```python
from build123d import *

# Parameters (mm, degrees)
DODANIE_WYCI_GNI_CIE1_DEPTH = 6
SZKIC3_R                    = 5.05
WYTNIJ_WYCI_GNI_CIE1_DEPTH  = 172.237795034
SZKIC5_R                    = 1.55
SZKIC5_W                    = 26
SZKIC5_H                    = 11
SZKIC5_W_2                  = 16
SZKIC5_H_2                  = 10
WYTNIJ_WYCI_GNI_CIE2_DEPTH  = 172.237795034
DODANIE_WYCI_GNI_CIE2_DEPTH = 6
SZKIC6_R                    = 1.55
WYTNIJ_WYCI_GNI_CIE3_DEPTH  = 172.237795034
DODANIE_WYCI_GNI_CIE3_DEPTH = 6
SZKIC9_R                    = 1.55
WYTNIJ_WYCI_GNI_CIE5_DEPTH  = 6
SZKIC11_R                   = 1.55
WYTNIJ_WYCI_GNI_CIE6_DEPTH  = 6
SZKIC15_R                   = 2.5
WYTNIJ_WYCI_GNI_CIE7_DEPTH  = 6
SZKIC8_R                    = 1.55
WYTNIJ_WYCI_GNI_CIE4_DEPTH  = 172.237795034
SZKIC20_W                   = 6.6
SZKIC20_H                   = 6.6
WYTNIJ_WYCI_GNI_CIE9_DEPTH  = 6
WYTNIJ_WYCI_GNI_CIE10_DEPTH = 10


with BuildPart() as part:
    # Szkic2 → Dodanie-wyciągnięcie1 (new body)
    with BuildSketch(Plane(origin=(0, 0, 0), x_dir=(1, 0, 0), z_dir=(0, 1, 0))):
        with BuildLine():
            Line((-2.705874152, 127.916025414), (-8.705874152, 127.916025414))
            ThreePointArc((-8.705874152, 127.916025414), (-10.120087715, 127.330238976), (-10.705874152, 125.916025414))
            Line((-10.705874152, 125.916025414), (-10.705874152, 88.696086508))
            ThreePointArc((-10.705874152, 88.696086508), (-11.877447027, 85.867659383), (-14.705874152, 84.696086508))
            Line((-14.705874152, 84.696086508), (-30.205874152, 84.696086508))
            ThreePointArc((-30.205874152, 84.696086508), (-33.034301277, 83.524513632), (-34.205874152, 80.696086508))
            Line((-34.205874152, 80.696086508), (-34.205874152, 69.929357434))
            Line((-34.205874152, 69.929357434), (-34.205874152, 68.036244156))
            Line((-34.205874152, 68.036244156), (-34.205874152, 10.604511111))
            Line((-34.205874152, 10.604511111), (-34.205874152, -19.154356935))
            ThreePointArc((-34.205874152, -19.154356935), (-21.880415638, -37.623287954), (-0.095732854, -33.328414665))
            Line((-0.095732854, -33.328414665), (14.157093559, -19.139859884))
            Line((14.157093559, -19.139859884), (55.027168237, 21.545915465))
            ThreePointArc((55.027168237, 21.545915465), (56.334805154, 23.495770338), (56.794125848, 25.798132784))
            Line((56.794125848, 25.798132784), (56.794125848, 30.935818421))
            Line((56.794125848, 30.935818421), (56.794125848, 59.333926751))
            ThreePointArc((56.794125848, 59.333926751), (64.677605901, 81.048439594), (85.935948442, 90.090131813))
            Line((85.935948442, 90.090131813), (91.371133341, 90.090131813))
            ThreePointArc((91.371133341, 90.090131813), (105.458816444, 95.925441216), (111.294125848, 110.013124319))
            Line((111.294125848, 110.013124319), (111.294125848, 128))
            ThreePointArc((111.294125848, 128), (110.70833941, 129.414213562), (109.294125848, 130))
            Line((109.294125848, 130), (103.294125848, 130))
            ThreePointArc((103.294125848, 130), (101.879912285, 129.414213562), (101.294125848, 128))
            Line((101.294125848, 128), (101.294125848, 110))
            ThreePointArc((101.294125848, 110), (98.36519366, 102.928932188), (91.294125848, 100))
            Line((91.294125848, 100), (9.294125848, 100))
            ThreePointArc((9.294125848, 100), (2.223058036, 102.928932188), (-0.705874152, 110))
            Line((-0.705874152, 110), (-0.705874152, 125.916025414))
            ThreePointArc((-0.705874152, 125.916025414), (-1.29166059, 127.330238976), (-2.705874152, 127.916025414))
        make_face()
    extrude(amount=DODANIE_WYCI_GNI_CIE1_DEPTH)

    # Szkic3 → Wytnij-wyciągnięcie1 (cut, through all)
    with BuildSketch(Plane(origin=(0, 6, 0), x_dir=(1, 0, 0), z_dir=(0, 1, 0))):
        with Locations(Location((-13.29618586, -25.303913492, 0), (0, 0, 270))):
            Circle(SZKIC3_R)
    extrude(amount=-WYTNIJ_WYCI_GNI_CIE1_DEPTH, mode=Mode.SUBTRACT)

    # Szkic5 → Wytnij-wyciągnięcie2 (cut, through all)
    with BuildSketch(Plane(origin=(0, 6, 0), x_dir=(1, 0, 0), z_dir=(0, 1, 0))):
        with Locations(Location((40.894125848, 75.45, 0), (0, 0, 270))):
            Circle(SZKIC5_R)
        with Locations(Location((30.260526652, 95, 0), (0, 0, 270))):
            Circle(SZKIC5_R)
        with Locations(Location((6.360542819, 95, 0), (0, 0, 270))):
            Circle(SZKIC5_R)
        with Locations(Location((40.894125848, 46.55, 0), (0, 0, 270))):
            Circle(SZKIC5_R)
        with Locations(Location((17.894125848, 72, 0), (0, 0, 270))):
            Circle(SZKIC5_R)
        with Locations((10.894125848, 52.5)):
            Rectangle(SZKIC5_W, SZKIC5_H)
        with Locations((15.894125848, 85)):
            Rectangle(SZKIC5_W_2, SZKIC5_H_2)
    extrude(amount=-WYTNIJ_WYCI_GNI_CIE2_DEPTH, mode=Mode.SUBTRACT)

    # Szkic12 → Dodanie-wyciągnięcie2 (add)
    with BuildSketch(Plane.XZ):
        with BuildLine():
            Line((28.406352316, 21.766792401), (22.674893132, 30.029606522))
            ThreePointArc((22.674893132, 30.029606522), (15.741620567, 36.230120828), (6.753517107, 38.623996834))
            Line((6.753517107, 38.623996834), (-1.505533921, 38.835570804))
            Line((-1.505533921, 38.835570804), (-13.693695858, 39.147797694))
            Line((-13.693695858, 39.147797694), (55.027168237, -21.545915465))
            ThreePointArc((55.027168237, -21.545915465), (56.334805154, -23.495770338), (56.794125848, -25.798132784))
            Line((56.794125848, -25.798132784), (56.794125848, -59.333926751))
            ThreePointArc((56.794125848, -59.333926751), (64.677605901, -81.048439594), (85.935948442, -90.090131813))
            Line((85.935948442, -90.090131813), (91.371133341, -90.090131813))
            Line((91.371133341, -90.090131813), (111.294125848, -110.013124319))
            Line((111.294125848, -110.013124319), (111.294125848, -103.986622655))
            ThreePointArc((111.294125848, -103.986622655), (110.381700995, -98.014648527), (107.72767835, -92.58757216))
            Line((107.72767835, -92.58757216), (89.166132072, -65.828137643))
            Line((89.166132072, -65.828137643), (62.775344571, -27.781601032))
            Line((62.775344571, -27.781601032), (28.406352316, 21.766792401))
        make_face()
    extrude(amount=-DODANIE_WYCI_GNI_CIE2_DEPTH)

    # Szkic6 → Wytnij-wyciągnięcie3 (cut, through all)
    with BuildSketch(Plane.XZ):
        with Locations(Location((68.241593591, -68.382704099, 0), (0, 0, 270))):
            Circle(SZKIC6_R)
    extrude(amount=-WYTNIJ_WYCI_GNI_CIE3_DEPTH, mode=Mode.SUBTRACT)

    # Szkic13 → Dodanie-wyciągnięcie3 (add)
    with BuildSketch(Plane.XZ):
        with BuildLine():
            Line((-34.205874152, -80.696086508), (-34.205874152, -90.183506419))
            ThreePointArc((-34.205874152, -90.183506419), (-33.840904211, -92.57229607), (-32.779295153, -94.743126617))
            Line((-32.779295153, -94.743126617), (-10.365682355, -127.055930463))
            ThreePointArc((-10.365682355, -127.055930463), (-9.649740147, -127.688003136), (-8.722327105, -127.916025414))
            Line((-8.722327105, -127.916025414), (-6.264571206, -127.916025414))
            Line((-6.264571206, -127.916025414), (-6.264571206, -80.696086508))
            Line((-6.264571206, -80.696086508), (-8.705874152, -80.696086508))
            Line((-8.705874152, -80.696086508), (-34.205874152, -80.696086508))
        make_face()
    extrude(amount=-DODANIE_WYCI_GNI_CIE3_DEPTH)

    # Szkic9 → Wytnij-wyciągnięcie5 (cut)
    with BuildSketch(Plane.XZ):
        with Locations(Location((63.668699873, -36.96490988, 0), (0, 0, 270))):
            Circle(SZKIC9_R)
    extrude(amount=-WYTNIJ_WYCI_GNI_CIE5_DEPTH, mode=Mode.SUBTRACT)

    # Szkic11 → Wytnij-wyciągnięcie6 (cut)
    with BuildSketch(Plane.XZ):
        with Locations(Location((-29.337186675, -72.387878859, 0), (0, 0, 270))):
            Circle(SZKIC11_R)
    extrude(amount=-WYTNIJ_WYCI_GNI_CIE6_DEPTH, mode=Mode.SUBTRACT)

    # Szkic15 → Wytnij-wyciągnięcie7 (cut)
    with BuildSketch(Plane.XZ):
        with Locations(Location((50.565790386, -80.001305928, 0), (0, 0, 270))):
            Circle(SZKIC15_R)
        with Locations(Location((50.484519469, -95.001085761, 0), (0, 0, 270))):
            Circle(SZKIC15_R)
    extrude(amount=-WYTNIJ_WYCI_GNI_CIE7_DEPTH, mode=Mode.SUBTRACT)

    # Szkic8 → Wytnij-wyciągnięcie4 (cut, through all)
    with BuildSketch(Plane.XZ):
        with Locations(Location((-19.205874152, -93.746086504, 0), (0, 0, 270))):
            Circle(SZKIC8_R)
    extrude(amount=-WYTNIJ_WYCI_GNI_CIE4_DEPTH, mode=Mode.SUBTRACT)

    # Szkic20 → Wytnij-wyciągnięcie9 (cut)
    with BuildSketch(Plane.XZ):
        with Locations((34.894125848, -26)):
            Rectangle(SZKIC20_W, SZKIC20_H)
        with Locations((-4.105874152, -89)):
            Rectangle(SZKIC20_W, SZKIC20_H)
    extrude(amount=-WYTNIJ_WYCI_GNI_CIE9_DEPTH, mode=Mode.SUBTRACT)

    # Szkic21 → Wytnij-wyciągnięcie10 (cut)
    with BuildSketch(Plane.XZ):
        with BuildLine():
            Line((62.051453687, -32.001592967), (61.640614874, -32.286569229))
            ThreePointArc((61.640614874, -32.286569229), (59.396767724, -32.773629702), (57.465724425, -31.531393928))
            Line((57.465724425, -31.531393928), (14.621138886, 30.235921359))
            ThreePointArc((14.621138886, 30.235921359), (7.68786632, 36.436435664), (-1.300237139, 38.830311671))
            Line((-1.300237139, 38.830311671), (6.753517107, 38.623996834))
            ThreePointArc((6.753517107, 38.623996834), (15.741620567, 36.230120828), (22.674893132, 30.029606522))
            Line((22.674893132, 30.029606522), (66.226344136, -32.756768268))
            ThreePointArc((66.226344136, -32.756768268), (64.295300837, -31.514532495), (62.051453687, -32.001592967))
        make_face()
    extrude(amount=-WYTNIJ_WYCI_GNI_CIE10_DEPTH, mode=Mode.SUBTRACT)


solid = part.part
```
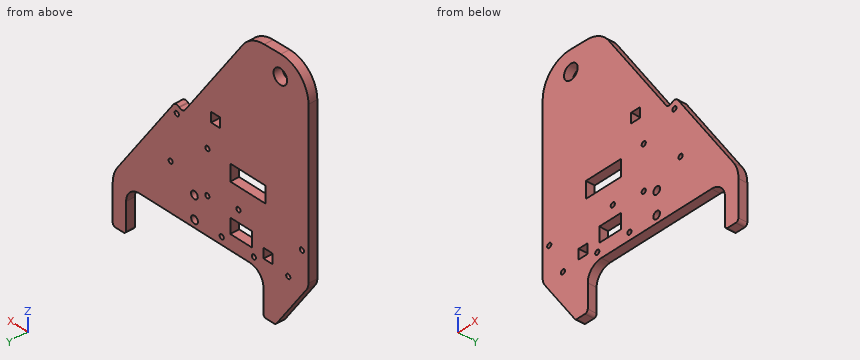
Input: part model. Units: mm. Frame: model coordinates. Give positions to 0.01 mm unless a question says otherwise; leave off trailing zeros. Order: outer loops, then holes, each group sorted by start corner. A loop starts at its lowest first (then second) coordinate and runs counter-clockwise, first axis right, second up. Notation, with made-up numbers: (44, -24.5) - (52, -24.5) arc R24 ccw to (52, -9.5) - close; hole circle Ø6 at (-13, 7). An arc over 180 degrees is marked (long way). One line per item, written item: value.
1. Cut plane B-B, the plane z = 26. Output: boundary loops of the cut face in (x, y).
Determined:
outline: (-33, 0) - (-18.3, 0) - (-18.3, 6) - (-33, 6) - close; (-8.29, 0) - (17.56, 0) - (17.56, 6) - (-8.29, 6) - close
2. Cut plane A-A, the plane x = 34.5. Output: boundary loops of the cut face in (y, z), and give its area (3 significant figures).
Determined:
outline: (0, -100) - (6, -100) - (6, -29.3) - (0, -29.3) - close; (0, -22.7) - (6, -22.7) - (6, 1.58) - (0, 1.58) - close
area: 570 mm2
3. Cut plane C-C, the plane z = -4.5. Output: boundary loops of the cut face in (x, y).
Determined:
outline: (-34.21, 0) - (38.72, 0) - (38.72, 6) - (-34.21, 6) - close
4. Cut plane D-D, the plane y = 1.55. Give the number of separate pieces and of enclosed holes in the cut face, and give its area (3 significant figures).
Determined:
separate pieces: 1
enclosed holes: 16
area: 13,200 mm2
5. Pin query (flat end, axial travel): pin 1 Ø1.8 at (x, y) = (13.5, 1.5) entering from -Z; pin 2 Ø12 at (x, z) = (19, -22) entering from -Y; pin 3 Ø1.9 at (x, z) = (6.36, -95) entering from +Y; pin 4 Ø1.8 at (x, y) = (33.5, 3) entering from +Z. Return the tip coordinate at first contact, or that it passes through.
Determined:
pin 1: z = -100
pin 2: y = 0
pin 3: through
pin 4: z = 4.32
6. Line query: probe 1 along Z at (x, y) = (-1, 5.25); probe 2 along Z at (x, y) = (6, 5.4); probe 3 along Z at (x, y) = (69.5, 4). Output: solid intervals per line, ascending.
Determined:
probe 1: -126.96 to -92.3, -85.7 to -58, -47 to 38.82
probe 2: -100.56 to -96.51, -93.49 to -58, -47 to 37.25
probe 3: -100 to -69.29, -67.48 to -37.48
